Input: part model. Units: mm. Frame: model coordinates. A direction names the side the tool comes from. Coordinates: 2 decimals unless noted, no trailing zeros. Write each loop counter-clockwise with the first axis right and the second up, starting at its lowest first coordinate (ties: lowest second). Pieces come first, ordered by that corner, then holes. Notation, with made-up numbers: (81.25, -10) - (85.25, -10) arc R20 cw to (85.25, 28) - close; hole circle Ø6 at (-10, -1.5). An arc over 180 degrees is marked (long way). One line per question, with ' | ' between items. Start each with the question number.
1) Section query B-B on z = 0. Return loops of the section in (x, y), and give its area (3 significant figures).
2) Section query D-D on x = 5.5. Return loops of the section in (y, z), and give its area (3 significant figures).
3) Draft query along Z for faces 1 (the cylindrical face through (22.5, 1, -0.1)), 2 (the flat face through (0, 1, 5)), 3 (the cylindrical face through (-0.54, 3.03, 2.44)). Return one class per face: released by +Z, released by -Z, zero draft, split by the parting line, or undercut.
4) Reachability of faces 4 (the flat face through (2, 5, 2)), 5 (the cylindrical face through (3.233, 3.479, -1.341)) from +Z, -Z, +X, -X, +Y, -Y: full face, straight path, thin tool, end or side. Return the list, or none.
5) First-contact query: P1, Ø2, axis at y = 4, z = -3, coming from the +X side; P2, Ø1, axis at x = -9.5, z = 4, coming from the +Y side; P3, Ø2.5, axis at x = 0, z = -1, coming from the +Y side. Flat tips, straight axial feed; report the tip coordinate or a pass-through.
6) Section query C-C on y = 3.9. Return loops of the section in (x, z).
7) Section query A-A on x = 0. Return loops of the section in (y, z), and give its area (3 significant figures).
8) Line query: line 1 (Z direction, x = 0, y = 3.8); line 2 (Y direction, x = -1, z = 4.75). Output: solid intervals per line, ascending.
Autodesk Inventor part; units mm, degrees
ref_plane "YZ Plane" through (0, 0, 0) normal (1, 0, 0) x (0, 1, 0)
ref_plane "XZ Plane" through (0, 0, 0) normal (0, 1, 0) x (-1, 0, 0)
ref_plane "XY Plane" through (0, 0, 0) normal (0, 0, 1) x (1, 0, 0)
sketch "Sketch1" plane through (0, 0, 0) normal (0, 1, 0) x (-1, 0, 0)
  line L0 (17.5, 0) -> (-17.5, 0) construction
  line L1 (17.5, 5) -> (-17.5, 5)
  line L2 (-17.5, -5) -> (17.5, -5)
  arc A0 (17.5, -5) -> (17.5, 5) centre (17.5, 0) ccw
  arc A1 (-17.5, 5) -> (-17.5, -5) centre (-17.5, 0) ccw
  point P0 (0, 0)
  dimension "d0" = 17.5
  dimension "d1" = 10
extrude "Extrusion1" add sketch "Sketch1" along normal blind 2
sketch "Sketch2" plane through (0, 2, 0) normal (0, 1, 0) x (1, 0, 0)
  circle A0 centre (0, 0) radius 3.5
  dimension "d4" = 7
extrude "Extrusion2" add sketch "Sketch2" along normal blind 3
sketch "Sketch3" plane through (0, 5, 0) normal (0, 1, 0) x (1, 0, 0)
  circle A0 centre (0, 0) radius 2.5
  point P0 (0, 0)
  dimension "d7" = 5
extrude "Extrusion3" cut sketch "Sketch3" against normal blind 4
properties part number "tang"
Answer key:
1) outline: (-22.5, 0) - (22.5, 0) - (22.5, 2) - (3.5, 2) - (3.5, 5) - (2.5, 5) - (2.5, 1) - (-2.5, 1) - (-2.5, 5) - (-3.5, 5) - (-3.5, 2) - (-22.5, 2) - close | area: 91.0 mm²
2) outline: (0, -5) - (2, -5) - (2, 5) - (0, 5) - close | area: 20.0 mm²
3) face 1: split by the parting line | face 2: released by +Z | face 3: undercut
4) face 4: +Z, -Z, +X, -X, +Y | face 5: +Y
5) P1: x = 2.87 | P2: y = 2 | P3: y = 1
6) outline: circle Ø7 at (0, 0); hole circle Ø5 at (0, 0)
7) outline: (0, -5) - (2, -5) - (2, -3.5) - (5, -3.5) - (5, -2.5) - (1, -2.5) - (1, 2.5) - (5, 2.5) - (5, 3.5) - (2, 3.5) - (2, 5) - (0, 5) - close | area: 21.0 mm²
8) line 1: -3.5 to -2.5, 2.5 to 3.5 | line 2: 0 to 2
